Input: part model. Units: mm. Frame: model coordinates. Face numbers are marked on the shaded views. A direction names the side the tool comes from. Coordinates: 2 decimals unless noted, no trailing zeros. Loops run counter-clockwise (first coordinate to the right, second up) from the corner with the lowest first, then second, coordinate; pieces in that order, holes last. Notation, with made-up numbers: M 86.5,19.25 L 99.5,19.25 A15 ccw 99.5,30.25 Z; hole C 48,77 d11. An arc over 180 degrees is marked long. Use a Markdown table: item, result. Add a question column.
1. Section A-A on x = 40.5. Output: boundary loops of the cut face in (y, z), then the cut area to 3 significant figures.
2. Section B-B on z = -6.75. Output: boundary loops of the cut face in (x, y).
3. Pin query (flat end, axial travel): pin 1 (2 mm diameter, centred on y = -9.5, z = -5, fed in from +X); pin 2 (1.5 mm diameter, centred on x = -93, z = -2, fed in from -Y); pin 3 (2 mm diameter, centred on x = 60, z = -6.5, fed in from +Y). Return the tip coordinate at first contact, or that it passes through.
4. Set-up query: the marked faces 1 and 2. Return all of +Z, -Z, +X, -X, +Y, -Y with unobstructed straight access to the full face (end or side cutting, diameter ignored); none if empty.
5. Section C-C on y = 7.75. Output: boundary loops of the cut face in (x, z), then the cut area to 3 significant figures.
6. Line query: L1, parallel to Z at x = -64, y = -7.75; L2, parallel to Y at x = -84.5, z = -4.5; L3, parallel to X at y = -11.5, z = -0.75. Output: solid intervals per line, ascending. Write a range as [from, to].
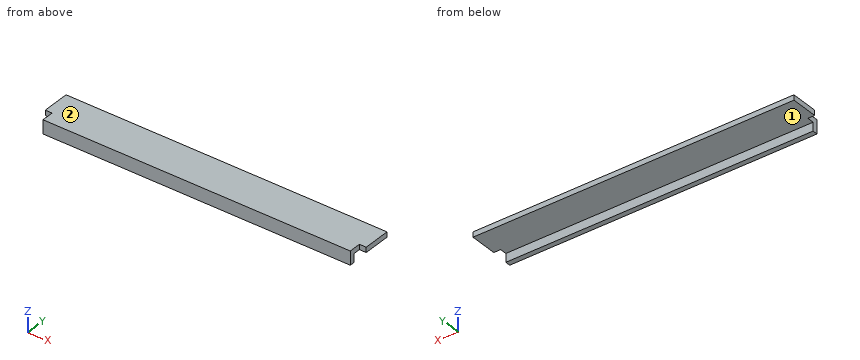
Solid Edge part; units mm, degrees
sketch "Sketch1" plane through (0, 0, 0) normal (0, 0, 1) x (1, 0, 0)
  line L0 (94, 10) -> (94, -10)
  line L1 (94, -10) -> (-94, -10)
  line L2 (-94, -10) -> (-94, 10)
  line L3 (-94, 10) -> (94, 10)
extrude "Protrusion1" add sketch "Sketch1" against normal blind 3
sketch "Sketch2" plane through (0, 0, 0) normal (0, 0, 1) x (1, 0, 0)
  line L0 (90, -13) -> (-90, -13)
  line L1 (-90, -13) -> (-90, -10)
  line L2 (-90, -10) -> (90, -10)
  line L3 (90, -10) -> (90, -13)
extrude "Protrusão_Extrudada_2" add sketch "Sketch2" against normal blind 8
sketch "Sketch3" plane through (0, -1.5, 0) normal (0, 0, 1) x (1, 0, 0)
  line L0 (90, -4.5) -> (94, -4.5)
  line L1 (94, -4.5) -> (94, -8.5)
  line L2 (94, -8.5) -> (90, -8.5)
  line L3 (90, -8.5) -> (90, -4.5)
  line L4 (-94, -8.5) -> (-90, -8.5)
  line L5 (-90, -8.5) -> (-90, -4.5)
  line L6 (-90, -4.5) -> (-94, -4.5)
  line L7 (-94, -4.5) -> (-94, -8.5)
extrude "Recorte_Extrudado_1" cut sketch "Sketch3" against normal blind 53.6894
Answers below:
| question | item | result |
|---|---|---|
| 1 | outline | M -13,-8 L -10,-8 L -10,-3 L 10,-3 L 10,0 L -13,0 Z |
| 1 | area | 84.0 mm² |
| 2 | outline | M -90,-13 L 90,-13 L 90,-10 L -90,-10 Z |
| 3 | pin 1 | stops at x = 90 |
| 3 | pin 2 | stops at y = -6 |
| 3 | pin 3 | stops at y = -10 |
| 4 | face 1 | -Z, +X, -X, +Y |
| 4 | face 2 | +Z, +X, -X, +Y, -Y |
| 5 | outline | M -94,-3 L 94,-3 L 94,0 L -94,0 Z |
| 5 | area | 564 mm² |
| 6 | L1 | z = [-3, 0] |
| 6 | L2 | y = [-13, -10] |
| 6 | L3 | x = [-90, 90] |
